Geometry check sheet. Reference: drawing and pictorial views, mm from the part's lowest x, y, z. Coordinates: 2 decimals unless noted, no trailing zeros. Loops run counter-clockwise (first coordinate to the right, second up) from the corner with the lowest first, then second, coordinate; pieces in that order, holes last. Notation, with made-up numbers: (-37.75, 21.25) - (-21.75, 21.25) arc R14 cw to (-21.75, 30.25) - close; hole circle Ø9 at (19.25, 4). An arc over 180 degrees is marked (long way). Write each question's results on one line, items separated by ' | '. Start each with the question number.
1. Cross-section at A-A (y = 25). Record the cut outline in (x, z), and give its area (3 significant figures).
2. Cross-section at B-B (x = 33). Record the cut outline in (y, z), and give its area (3 significant figures).
3. Cross-section at C-C (x = 11.5). Record the cut outline in (y, z) (1 decimal).
4. Gauge pin test, flat ends, axial feed: P1, Ø1, axis at x = 21, z = 1.5, coming from the -Y side; P2, Ø2, axis at x = 25, y = 37.5, coming from the +Z side; P3, Ø3, axis at x = 13.5, z = 4, coming from the +Y side. Record the tip position at first contact, or that the pin passes through.
5. Cross-section at D-D (z = 0.6). Give the number of separate pieces and of enclosed holes in the cut face, and give its area (3 significant figures).
6. Draft check along Y on the marked faces 1, 2 and 3. Enter one of: released by +Y, released by -Y, zero draft, split by the parting line, or undercut.
7. Thickness scan on line 1 (Y direction, x = 25, z = 3.75); line 2 (Y direction, x = 40, z = 3.4) (1 decimal); line 3 (X direction, y = 11, z = 0.5) (1 decimal). Record the ranges inside material, lowest first. Write a range as [from, to].
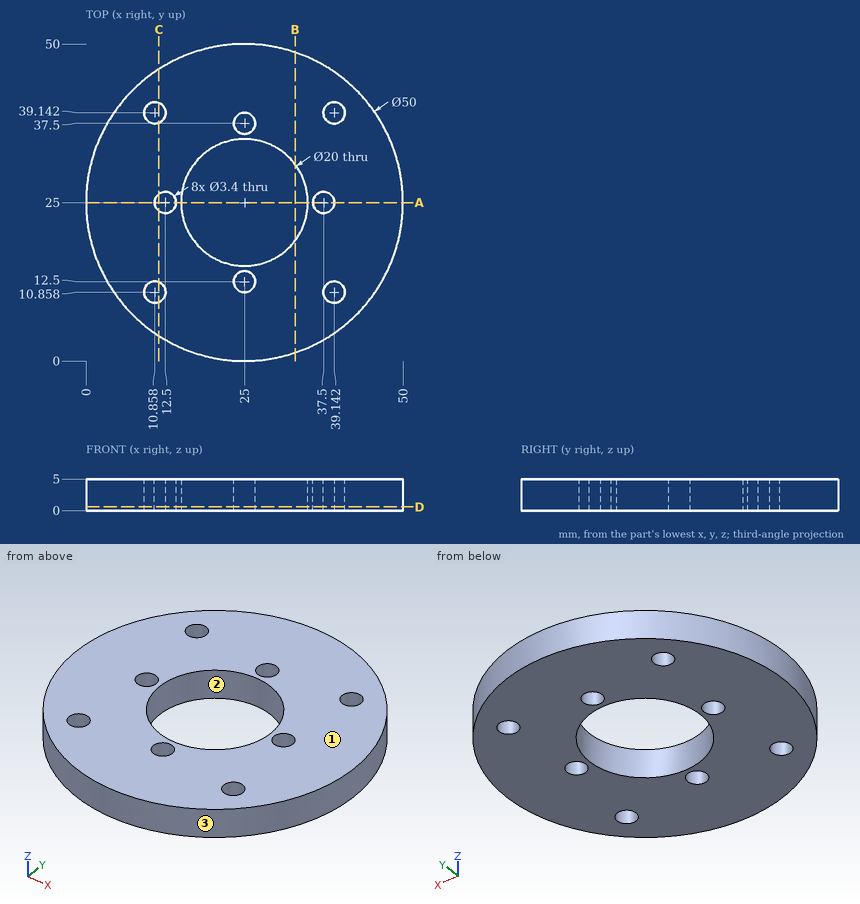
Established:
1) outline: (0, 0) - (10.8, 0) - (10.8, 5) - (0, 5) - close; (14.2, 0) - (15, 0) - (15, 5) - (14.2, 5) - close; (35, 0) - (35.8, 0) - (35.8, 5) - (35, 5) - close; (39.2, 0) - (50, 0) - (50, 5) - (39.2, 5) - close | area: 116 mm^2
2) outline: (1.31, 0) - (19, 0) - (19, 5) - (1.31, 5) - close; (31, 0) - (48.69, 0) - (48.69, 5) - (31, 5) - close | area: 177 mm^2
3) outline: (4, 0) - (9.3, 0) - (9.3, 5) - (4, 5) - close; (12.4, 0) - (23.6, 0) - (23.6, 5) - (12.4, 5) - close; (26.4, 0) - (37.6, 0) - (37.6, 5) - (26.4, 5) - close; (40.7, 0) - (46, 0) - (46, 5) - (40.7, 5) - close
4) P1: y = 0.25 | P2: through | P3: y = 47.91
5) separate pieces: 1 | enclosed holes: 9 | area: 1,580 mm^2
6) face 1: zero draft | face 2: undercut | face 3: split by the parting line
7) line 1: [0, 10.8], [14.2, 15], [35, 35.8], [39.2, 50] | line 2: [5, 9.4], [12.3, 37.7], [40.6, 45] | line 3: [4.3, 9.2], [12.6, 24.2], [25.8, 37.4], [40.8, 45.7]
